Check sheet for the modelled part. Datum: model origin and axes. Units: mm. A direction names the side the tool comes from. Give positions to 0.01 mm unless a question says otherwise; leave off trailing zeros. Write each loop counter-clockwise with the first axis right and the second up, starting at its lowest first coordinate (ties: lowest second). Pieces come first, ordered by that corner, then holes. Notation, with made-up numbers: M -26.75,-29 L -20.75,-29 A16 cw -20.75,-14 Z; hole C 41,36 d1. An arc over 180 degrees is marked long. One line per item, written item: value. Start each with the question number.
from build123d import *

# Parameters (mm, degrees)
F0_W     = 40
F0_H     = 40
F1_DEPTH = 10
F2_DEPTH = 5
F3_R     = 2
F4_DEPTH = 10


with BuildPart() as f1:
    # F0 (on Top) → F1 (new body)
    with BuildSketch(Plane.XY):
        Rectangle(F0_W, F0_H)
        with BuildLine():
            Line((-15, -12.5), (-15, 12.5))
            ThreePointArc((-15, 12.5), (-13.535534, 16.035534), (-10, 17.5))
            ThreePointArc((-10, 17.5), (-6.464466, 16.035534), (-5, 12.5))
            Line((-5, 12.5), (-5, -12.5))
            ThreePointArc((-5, -12.5), (-6.464466, -16.035534), (-10, -17.5))
            ThreePointArc((-10, -17.5), (-13.535534, -16.035534), (-15, -12.5))
        make_face(mode=Mode.SUBTRACT)
        with BuildLine():
            Line((5, -12.5), (5, 12.5))
            ThreePointArc((5, 12.5), (6.464466, 16.035534), (10, 17.5))
            ThreePointArc((10, 17.5), (13.535534, 16.035534), (15, 12.5))
            Line((15, 12.5), (15, -12.5))
            ThreePointArc((15, -12.5), (13.535534, -16.035534), (10, -17.5))
            ThreePointArc((10, -17.5), (6.464466, -16.035534), (5, -12.5))
        make_face(mode=Mode.SUBTRACT)
        with BuildLine():
            ThreePointArc((-10, 17.5), (-13.535534, 16.035534), (-15, 12.5))
            Line((-15, 12.5), (-15, -12.5))
            ThreePointArc((-15, -12.5), (-13.535534, -16.035534), (-10, -17.5))
            ThreePointArc((-10, -17.5), (-6.464466, -16.035534), (-5, -12.5))
            Line((-5, -12.5), (-5, 12.5))
            ThreePointArc((-5, 12.5), (-6.464466, 16.035534), (-10, 17.5))
        make_face()
        with BuildLine():
            ThreePointArc((-10, 15), (-8.232233, 14.267767), (-7.5, 12.5))
            Line((-7.5, 12.5), (-7.5, -12.5))
            ThreePointArc((-7.5, -12.5), (-8.232233, -14.267767), (-10, -15))
            ThreePointArc((-10, -15), (-11.767767, -14.267767), (-12.5, -12.5))
            Line((-12.5, -12.5), (-12.5, 12.5))
            ThreePointArc((-12.5, 12.5), (-11.767767, 14.267767), (-10, 15))
        make_face(mode=Mode.SUBTRACT)
        with BuildLine():
            ThreePointArc((10, 17.5), (6.464466, 16.035534), (5, 12.5))
            Line((5, 12.5), (5, -12.5))
            ThreePointArc((5, -12.5), (6.464466, -16.035534), (10, -17.5))
            ThreePointArc((10, -17.5), (13.535534, -16.035534), (15, -12.5))
            Line((15, -12.5), (15, 12.5))
            ThreePointArc((15, 12.5), (13.535534, 16.035534), (10, 17.5))
        make_face()
        with BuildLine():
            Line((7.5, -12.5), (7.5, 12.5))
            ThreePointArc((7.5, 12.5), (8.232233, 14.267767), (10, 15))
            ThreePointArc((10, 15), (11.767767, 14.267767), (12.5, 12.5))
            Line((12.5, 12.5), (12.5, -12.5))
            ThreePointArc((12.5, -12.5), (11.767767, -14.267767), (10, -15))
            ThreePointArc((10, -15), (8.232233, -14.267767), (7.5, -12.5))
        make_face(mode=Mode.SUBTRACT)
    extrude(amount=-F1_DEPTH)

    # F0 (on Top) → F2 (cut)
    with BuildSketch(Plane.XY):
        with BuildLine():
            Line((-7.5, -12.5), (-7.5, 12.5))
            ThreePointArc((-7.5, 12.5), (-8.232233, 14.267767), (-10, 15))
            ThreePointArc((-10, 15), (-11.767767, 14.267767), (-12.5, 12.5))
            Line((-12.5, 12.5), (-12.5, -12.5))
            ThreePointArc((-12.5, -12.5), (-11.767767, -14.267767), (-10, -15))
            ThreePointArc((-10, -15), (-8.232233, -14.267767), (-7.5, -12.5))
        make_face()
        with BuildLine():
            ThreePointArc((10, 15), (8.232233, 14.267767), (7.5, 12.5))
            Line((7.5, 12.5), (7.5, -12.5))
            ThreePointArc((7.5, -12.5), (8.232233, -14.267767), (10, -15))
            ThreePointArc((10, -15), (11.767767, -14.267767), (12.5, -12.5))
            Line((12.5, -12.5), (12.5, 12.5))
            ThreePointArc((12.5, 12.5), (11.767767, 14.267767), (10, 15))
        make_face()
        with BuildLine():
            ThreePointArc((10, 17.5), (6.464466, 16.035534), (5, 12.5))
            Line((5, 12.5), (5, -12.5))
            ThreePointArc((5, -12.5), (6.464466, -16.035534), (10, -17.5))
            ThreePointArc((10, -17.5), (13.535534, -16.035534), (15, -12.5))
            Line((15, -12.5), (15, 12.5))
            ThreePointArc((15, 12.5), (13.535534, 16.035534), (10, 17.5))
        make_face()
        with BuildLine():
            Line((7.5, -12.5), (7.5, 12.5))
            ThreePointArc((7.5, 12.5), (8.232233, 14.267767), (10, 15))
            ThreePointArc((10, 15), (11.767767, 14.267767), (12.5, 12.5))
            Line((12.5, 12.5), (12.5, -12.5))
            ThreePointArc((12.5, -12.5), (11.767767, -14.267767), (10, -15))
            ThreePointArc((10, -15), (8.232233, -14.267767), (7.5, -12.5))
        make_face(mode=Mode.SUBTRACT)
        with BuildLine():
            ThreePointArc((-10, 17.5), (-13.535534, 16.035534), (-15, 12.5))
            Line((-15, 12.5), (-15, -12.5))
            ThreePointArc((-15, -12.5), (-13.535534, -16.035534), (-10, -17.5))
            ThreePointArc((-10, -17.5), (-6.464466, -16.035534), (-5, -12.5))
            Line((-5, -12.5), (-5, 12.5))
            ThreePointArc((-5, 12.5), (-6.464466, 16.035534), (-10, 17.5))
        make_face()
        with BuildLine():
            ThreePointArc((-10, 15), (-8.232233, 14.267767), (-7.5, 12.5))
            Line((-7.5, 12.5), (-7.5, -12.5))
            ThreePointArc((-7.5, -12.5), (-8.232233, -14.267767), (-10, -15))
            ThreePointArc((-10, -15), (-11.767767, -14.267767), (-12.5, -12.5))
            Line((-12.5, -12.5), (-12.5, 12.5))
            ThreePointArc((-12.5, 12.5), (-11.767767, 14.267767), (-10, 15))
        make_face(mode=Mode.SUBTRACT)
    extrude(amount=-F2_DEPTH, mode=Mode.SUBTRACT)

    # F3 (on face) → F4 (cut)
    with BuildSketch(Plane.XZ.offset(20)):
        with Locations((0, -5)):
            Circle(F3_R)
    extrude(amount=-F4_DEPTH, mode=Mode.SUBTRACT)


solid = f1.part
1) Cross-section at D-D (x = 0). Record the boundary of the cut face in (y, z), plus the area to 3 significant figures.
2) Gauge pin test, flat ends, axial feed: pin 1 (8 mm diameter, centred on x = 10, y = -1.5, fed in from +Z); pin 2 (1 mm diameter, centred on x = -9.5, y = 5.5, fed in from +Z). Record the tip position at first contact, or that the pin passes through.
3) Cross-section at B-B (z = -0.75). Record the boundary of the cut face in (x, y).
4) Cross-section at C-C (x = -11.5). Record the boundary of the cut face in (y, z).
5) Draft check along Z on faces 1 (the flat face through (15, 0, -2)), 2 (the cylindrical face through (0, -15, -7)), 3 (the flat face through (-13, 0, -5)). Enter one of: released by +Z, released by -Z, zero draft, split by the parting line, or undercut.
6) Tool access check on faces 4 (the flat face through (0, -10, -5)), 5 (the flat face through (-7.5, 0, -7)), 6 (the flat face through (-5, 0, -2)). Record the directions out of +Z, -Z, +X, -X, +Y, -Y that give a thin tool (end or side, any length) a straight path to the whole face; none if there is none.
7) Material ranges on L1, parallel to X at y = 4, z = -4.5; L2, parallel to X at y = -9.5, z = -5.5; L3, parallel to Z at x = 0, y = -14, recorded low to high. Write a range as from..to.
8) Cross-section at A-A (y = 0.5). Record the boundary of the cut face in (x, z), plus the area to 3 significant figures.
Data:
1. outline: M -20,-10 L 20,-10 L 20,0 L -20,0 L -20,-3 L -10,-3 L -10,-7 L -20,-7 Z
1. area: 360 mm2
2. pin 1: stops at z = -5
2. pin 2: passes through
3. outline: M -20,-20 L 20,-20 L 20,20 L -20,20 Z; hole M -15,-12.5 A5 ccw -5,-12.5 L -5,12.5 A5 ccw -15,12.5 Z; hole M 5,-12.5 A5 ccw 15,-12.5 L 15,12.5 A5 ccw 5,12.5 Z
4. outline: M -20,-10 L -14.5,-10 L -14.5,-5 L -17.27,-5 L -17.27,0 L -20,0 Z; M 14.5,-10 L 20,-10 L 20,0 L 17.27,0 L 17.27,-5 L 14.5,-5 Z
5. face 1: zero draft
5. face 2: undercut
5. face 3: released by +Z
6. face 4: -Y
6. face 5: +Z, -Z
6. face 6: +Z
7. L1: x = -20..-15, -5..5, 15..20
7. L2: x = -20..-12.5, -7.5..7.5, 12.5..20
7. L3: z = -10..-7, -3..0
8. outline: M -20,-10 L -12.5,-10 L -12.5,-5 L -15,-5 L -15,0 L -20,0 Z; M -7.5,-10 L 7.5,-10 L 7.5,-5 L 5,-5 L 5,0 L -5,0 L -5,-5 L -7.5,-5 Z; M 12.5,-10 L 20,-10 L 20,0 L 15,0 L 15,-5 L 12.5,-5 Z
8. area: 250 mm2
